Design review of the part built by this model. Coordinates are the model's own, in mm. A direction names the side the tool comes from. Coordinates: 2 decimals unless noted, no trailing zeros. Order: outer loops, then holes, each group sorted by start corner. A loop starts at its lowest first (then second) coordinate and runs counter-clockwise, first axis right, second up. Notation, with made-up numbers: (53, 35) -> (92, 35) arc R30 ccw to (92, 65) -> close; hole circle Ø2 at (-4.75, 59.5). An arc over 180 degrees is marked (long way). Use a Markdown table: item, result. Add a question column.
Q1. Wall thickness on probe 1 along Y at (x, z) = (-254.5, -7); probe 2 along X at (y, z) = (124.5, -12.5); probe 3 along X at (y, z) = (179, -9.5): over which ranges is each line inside the solid? List them lowest first.
Q2. Add section A-A (x = -355.5). State the section outline as (y, z) points, then the cut area to 3 significant figures.
Q3. Machinability: for faces 4 (the face through (-296.694, 151.872, -8.041)), 5 (the face through (202.8, 152.1, -8)), which of the approach directions +Z, -Z, +X, -X, +Y, -Y give a long, thin tool a straight path to every point of the face, cutting with its end or side? Answer none if there is none.
Q4. Add section B-B (y = 214). State the section outline as (x, z) points, then the cut area to 3 significant figures.
Q5. Insertion check: pin 1 (1.5 mm diameter, centred on y = 187, z = -7.5, fed in from +X); pin 2 (6 mm diameter, centred on y = 61, z = -14.5, fed in from +X); pin 3 (8 mm diameter, centred on x = -600.5, z = -8, fed in from -Y) (3 decimals). Each pin has a flat end and moves straight along its axis. Give the tip position at first contact, or say it passes through.
Q6. Add section C-C (x = -609.5). State the section outline as (y, z) points (1 decimal).
Q7. The part is to be moulded in two halves that separate along Y. For faces 1 (the face through (-242, 240, 0)), 2 (the face through (-597.2, 147.9, -8)), 3 (the face through (-102.11, 148.13, -8.04)), say which applies: pulls with the +Y half, pulls with the -Y half, needs draft (parallel to the pull), parting line crosses it, or undercut.
Q8. Add section D-D (z = -10.5). Count the separate pieces of the cut face and the enclosed holes in it, then the cut area to 3 significant figures.
from build123d import *

# Parameters (mm, degrees)
BOSS_EXTRUDE1_DEPTH = 16.31
CUT_EXTRUDE4_DEPTH  = 130.31
SKETCH3_R           = 7.316006069
SKETCH3_R_2         = 6.6
CUT_EXTRUDE6_DEPTH  = 130.31


with BuildPart() as part:
    # Sketch1 → Boss-Extrude1 (new body)
    with BuildSketch(Plane.XY):
        Polygon((-800, 300), (400, 300), (0, 0), (-400, 0), align=None)
        Polygon((-394.563333333, 16.31), (-5.436666667, 16.31), (-201.528049499, 283.69), align=None, mode=Mode.SUBTRACT)
    extrude(amount=-BOSS_EXTRUDE1_DEPTH)

    # Sketch2 → Cut-Extrude4 (cut)
    with BuildSketch(Plane.XY):
        Polygon((-181.30202164, 283.69), (10.873333333, 26.546261845), (351.07, 283.69), align=None)
        Polygon((-751.07, 283.69), (-222.488676184, 283.69), (-412.777952758, 29.970964568), align=None)
    extrude(amount=-CUT_EXTRUDE4_DEPTH, mode=Mode.SUBTRACT)

    # Sketch3 → Cut-Extrude6 (cut)
    with BuildSketch(Plane.XY):
        with Locations((-200.996317691, 291.556411045)):
            Circle(SKETCH3_R)
        with Locations((-763.369850402, 286.770824774)):
            Circle(SKETCH3_R_2)
        with Locations((364.965045825, 286.770824774)):
            Circle(SKETCH3_R_2)
        with Locations((2.613340708, 20.373189048)):
            Circle(SKETCH3_R_2)
        with Locations((-406.577807344, 20.373189048)):
            Circle(SKETCH3_R_2)
    extrude(amount=-CUT_EXTRUDE6_DEPTH, mode=Mode.SUBTRACT)


solid = part.part
Established:
| question | item | result |
|---|---|---|
| 1 | probe 1 | 0 to 16.31, 210.32 to 241.01, 283.69 to 300 |
| 1 | probe 2 | -566 to -538.82, -341.88 to -316.46, -84.78 to -62.33, 140.46 to 166 |
| 1 | probe 3 | -638.67 to -611.48, -301.01 to -277.11, -124.75 to -103.06, 212.57 to 238.67 |
| 2 | outline | (0, -16.31) -> (16.31, -16.31) -> (16.31, 0) -> (0, 0) -> close; (70.42, -16.31) -> (106.34, -16.31) -> (106.34, 0) -> (70.42, 0) -> close; (283.69, -16.31) -> (300, -16.31) -> (300, 0) -> (283.69, 0) -> close |
| 2 | area | 1,120 mm^2 |
| 3 | face 4 | +Z, -Z |
| 3 | face 5 | +Z, -Z, +X, -Y |
| 4 | outline | (-685.33, -16.31) -> (-658.15, -16.31) -> (-658.15, 0) -> (-685.33, 0) -> close; (-274.76, -16.31) -> (-251.84, -16.31) -> (-251.84, 0) -> (-274.76, 0) -> close; (-150.42, -16.31) -> (-129.22, -16.31) -> (-129.22, 0) -> (-150.42, 0) -> close; (258.87, -16.31) -> (285.33, -16.31) -> (285.33, 0) -> (258.87, 0) -> close |
| 4 | area | 1,590 mm^2 |
| 5 | pin 1 | x = 250.33 |
| 5 | pin 2 | x = 85.33 |
| 5 | pin 3 | y = 147.375 |
| 6 | outline | (157.1, -16.3) -> (177.5, -16.3) -> (177.5, 0) -> (157.1, 0) -> close; (283.7, -16.3) -> (300, -16.3) -> (300, 0) -> (283.7, 0) -> close |
| 7 | face 1 | needs draft |
| 7 | face 2 | pulls with the -Y half |
| 7 | face 3 | undercut |
| 8 | separate pieces | 1 |
| 8 | enclosed holes | 8 |
| 8 | area | 51,800 mm^2 |
